Verification items for the finished model (mm, model axes). Face numbers are marked on the shaded views. A direction names the side the tool comes from. Coordinates: 2 decimals unless noted, no trailing zeros. Order: outer loops, then holes, each group sorted by start corner. A loop starts at its lowest first (then second) coordinate and runs counter-clockwise, first axis right, second up. Notation, with made-up numbers: M 37.5,12 L 56.5,12 A22 cw 56.5,50 Z; hole C -19.75,-16.5 d3. An arc over 180 degrees is marked long. Return JSON: item names as keys, results as strings. Group by question number.
1. Section check C-C, the plane y = 15. Record the cut outline in (x, z), plus the area to 3 significant figures.
2. Set-up check for the marked faces 1 and 2: record each of +Z, -Z, +X, -X, +Y, -Y from which the full face is reachable in a straight line by a thin tool's end or side.
3. Gauge pin test, flat ends, axial feed: pin 1 (5 mm diameter, centred on x = 19, z = 15, fed in from +Y); pin 2 (1.5 mm diameter, centred on x = 39, y = 38.5, fed in from +Z). Record the tip position at first contact, or that the pin passes through.
4. Section check A-A, the plane z = 14. Record the cut outline in (x, y), plus the area to 3 significant figures.
5. Section check B-B, the plane x = 28. Record the cut outline in (y, z), plus the area to 3 significant figures.
6. Material ranges on line 1 along Z through (x, y) = (6.5, 4); line 2 along X through (y, z) = (19, 20.5); line 3 along X through (y, z) = (16, 25.25), recorded low to high.
7. Mould release check, pull along Z, two halves, no side actions. Record for the marked faces 3, 4 and 5: +Z half, -Z half, draft (parallel to the pull), parting line (faces both ways), or undercut.
8. Section check D-D, the plane x = 43.5. Record the cut outline in (y, z).
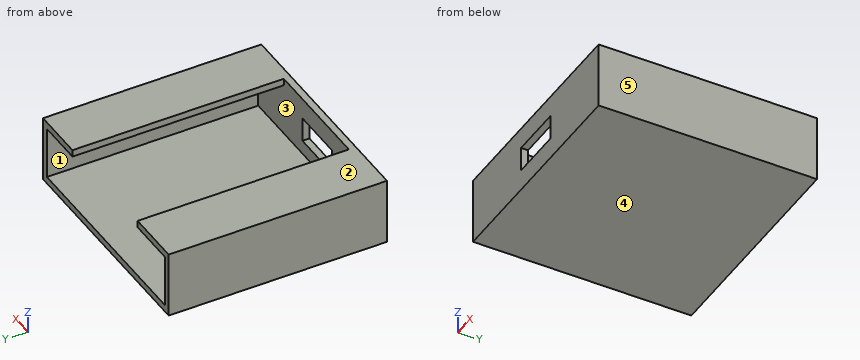
```python
from build123d import *

# Parameters (mm, degrees)
F0_W     = 15
F0_H     = 7
F1_DEPTH = 2
F2_DEPTH = 60


with BuildPart() as f1:
    # F0 (on Front) → F1 (new body)
    with BuildSketch(Plane.XZ):
        Polygon((0, 23.638431), (0, 8.638419), (60, 8.638419), (60, 23.638419), (46.979439, 23.638419), (46.979439, 25.643766), (13.85323, 25.643766), (13.85323, 23.638431), align=None)
        with Locations((30, 16.138419)):
            Rectangle(F0_W, F0_H, mode=Mode.SUBTRACT)
        Polygon((60, 8.638419), (0, 8.638419), (0, 23.638431), (13.85323, 23.638431), (13.85323, 25.643766), (-1.963923, 25.643766), (-1.963923, 6.638419), (61.979439, 6.638419), (61.979439, 25.643766), (46.979439, 25.643766), (46.979439, 23.638419), (60, 23.638419), align=None)
    extrude(amount=F1_DEPTH)

    # F0 (on Front) → F2 (join)
    with BuildSketch(Plane.XZ):
        Polygon((60, 8.638419), (0, 8.638419), (0, 23.638431), (13.85323, 23.638431), (13.85323, 25.643766), (-1.963923, 25.643766), (-1.963923, 6.638419), (61.979439, 6.638419), (61.979439, 25.643766), (46.979439, 25.643766), (46.979439, 23.638419), (60, 23.638419), align=None)
    extrude(amount=-F2_DEPTH)


solid = f1.part
```
Answers follow:
{
 "1": {"outline": "M -1.96,6.64 L 61.98,6.64 L 61.98,25.64 L 46.98,25.64 L 46.98,23.64 L 60,23.64 L 60,8.64 L 0,8.64 L 0,23.64 L 13.85,23.64 L 13.85,25.64 L -1.96,25.64 Z", "area": "249 mm^2"},
 "2": {"face 1": "+Y", "face 2": "+Z, +X, -X, +Y, -Y"},
 "3": {"pin 1": "y = 0", "pin 2": "z = 8.64"},
 "4": {"outline": "M -1.96,-2 L 22.5,-2 L 22.5,0 L 0,0 L 0,60 L -1.96,60 Z; M 37.5,-2 L 61.98,-2 L 61.98,60 L 60,60 L 60,0 L 37.5,0 Z", "area": "334 mm^2"},
 "5": {"outline": "M -2,6.64 L 60,6.64 L 60,8.64 L 0,8.64 L 0,12.64 L -2,12.64 Z; M -2,19.64 L 0,19.64 L 0,25.64 L -2,25.64 Z", "area": "144 mm^2"},
 "6": {"line 1": "6.64 to 8.64, 23.64 to 25.64", "line 2": "-1.96 to 0, 60 to 61.98", "line 3": "-1.96 to 13.85, 46.98 to 61.98"},
 "7": {"face 3": "undercut", "face 4": "-Z half", "face 5": "draft"},
 "8": {"outline": "M -2,6.64 L 60,6.64 L 60,8.64 L 0,8.64 L 0,25.64 L -2,25.64 Z"}
}
